from build123d import *

# Parameters (mm, degrees)
SKETCH1_W           = 18
SKETCH1_H           = 3.78
BOSS_EXTRUDE1_DEPTH = 0.5
BOSS_EXTRUDE2_DEPTH = 3.2
SKETCH4_W           = 4
SKETCH4_H           = 3.78
CUT_EXTRUDE1_DEPTH  = 0.8
FILLET1_R           = 4.5


with BuildPart() as part:
    # Sketch1 → Boss-Extrude1 (new body)
    with BuildSketch(Plane.XY):
        Rectangle(SKETCH1_W, SKETCH1_H)
    extrude(amount=BOSS_EXTRUDE1_DEPTH)

    # Sketch3 → Boss-Extrude2 (add)
    with BuildSketch(Plane.XY.offset(0.5)):
        with BuildLine():
            Line((-3.825, -1.89), (3.825, -1.89))
            ThreePointArc((3.825, -1.89), (4.532106781, -1.597106781), (4.825, -0.89))
            Line((4.825, -0.89), (4.825, 0.89))
            ThreePointArc((4.825, 0.89), (4.532106781, 1.597106781), (3.825, 1.89))
            Line((3.825, 1.89), (-3.825, 1.89))
            ThreePointArc((-3.825, 1.89), (-4.532106781, 1.597106781), (-4.825, 0.89))
            Line((-4.825, 0.89), (-4.825, -0.89))
            ThreePointArc((-4.825, -0.89), (-4.532106781, -1.597106781), (-3.825, -1.89))
        make_face()
    extrude(amount=BOSS_EXTRUDE2_DEPTH)

    # Sketch4 → Cut-Extrude1 (cut)
    with BuildSketch(Plane(origin=(0, 0, 0), x_dir=(-1, 0, 0), z_dir=(0, 0, -1))):
        Rectangle(SKETCH4_W, SKETCH4_H)
    extrude(amount=-CUT_EXTRUDE1_DEPTH, mode=Mode.SUBTRACT)

    # Fillet1
    # the kernel refuses this fillet: 4.5 mm, written as the material it takes off along each edge
    with BuildSketch(Plane(origin=(-2, -8.293124237, 0), x_dir=(-1, 0, 0), z_dir=(0, 1, 0))) as fillet1_piece_1:
        with BuildLine():
            CenterArc((2.561249695, 4.5), FILLET1_R, 235.307869415, 34.692130585)
            Line((0, 0.8), (-0.051224994, 0.726))
            ThreePointArc((-0.051224994, 0.726), (-0.09, 0.4), (-0.09, 0))
            Line((-0.09, 0), (0, -0.09))
            Line((0, -0.09), (2.561249695, -0.09))
            Line((2.561249695, -0.09), (2.561249695, 0))
        make_face()
    extrude(amount=16.586248475, mode=Mode.SUBTRACT)
    with BuildSketch(Plane(origin=(2, 8.293124237, 0), x_dir=(1.0735856648108615e-12, 0, 1.0), z_dir=(0, -1, 0))) as fillet1_piece_2:
        with BuildLine():
            CenterArc((4.5, -2.561249695), FILLET1_R, 145.307869415, 34.692130585)
            Line((0, -2.561249695), (-0.09, -2.561249695))
            Line((-0.09, -2.561249695), (-0.09, 0))
            Line((-0.09, 0), (0, 0.09))
            ThreePointArc((0, 0.09), (0.4, 0.09), (0.726, 0.051224994))
            Line((0.726, 0.051224994), (0.8, 0))
        make_face()
    extrude(amount=16.586248475, mode=Mode.SUBTRACT)


solid = part.part
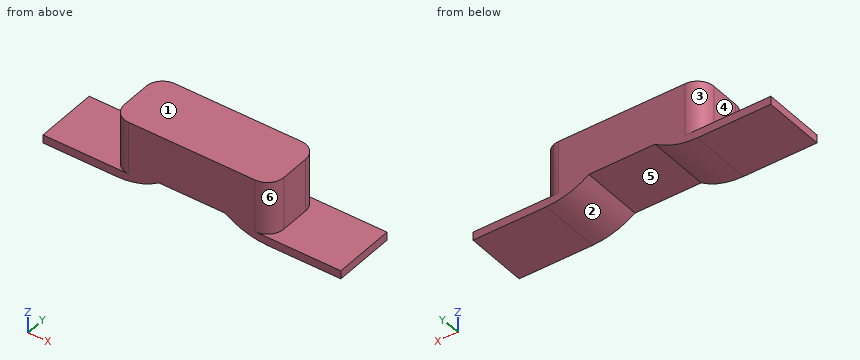
Verification items for the finished model (mm, model axes). Face numbers are marked on the shaded views. A direction names the side the tool comes from. Coordinates: 2 decimals unless noted, no trailing zeros. Order: outer loops, then holes, each group sorted by start corner. A loop starts at its lowest first (then second) coordinate and runs counter-clockwise, first axis right, second up.
Item 1: Access from +Z, -Z, +X, -X, +Y, -Y to the whole of each face (thin tool, end or side, straight path). Record for the marked faces 4, 5 and 6.
Filled in:
face 4: +Z, -X, +Y, -Y
face 5: -Z, +Y, -Y
face 6: +Z, +X, -Y
Item 2: Section check C-C, the plane x = -5.25. Enter the section's corners in (y, z), then the cut area to 3 significant figures.
Filled in:
outline: (-1.89, 0) - (1.89, 0) - (1.89, 0.5) - (-1.89, 0.5) - close
area: 1.89 mm2
Item 3: Section check D-D, the plane y = -1.1. Enter the section's corners in (x, z), then the cut area to 3 significant figures.
Filled in:
outline: (-9, 0) - (-4.56, 0) arc R4.5 ccw to (-2, 0.8) - (2, 0.8) arc R4.5 ccw to (4.56, 0) - (9, 0) - (9, 0.5) - (4.8, 0.5) - (4.8, 3.7) - (-4.8, 3.7) - (-4.8, 0.5) - (-9, 0.5) - close
area: 35.2 mm2
Item 4: Section check A-A, the plane z = 1.7. Enter the section's corners in (x, y) (3 decimals), then the cut area to 3 significant figures.
Filled in:
outline: (-4.825, -0.89) arc R1 ccw to (-3.825, -1.89) - (3.825, -1.89) arc R1 ccw to (4.825, -0.89) - (4.825, 0.89) arc R1 ccw to (3.825, 1.89) - (-3.825, 1.89) arc R1 ccw to (-4.825, 0.89) - close
area: 35.6 mm2
Item 5: Section check B-B, the plane y = 0.3. Enter the section's corners in (x, z) (3 decimals).
Filled in:
outline: (-9, 0) - (-4.561, 0) arc R4.5 ccw to (-2, 0.8) - (2, 0.8) arc R4.5 ccw to (4.561, 0) - (9, 0) - (9, 0.5) - (4.825, 0.5) - (4.825, 3.7) - (-4.825, 3.7) - (-4.825, 0.5) - (-9, 0.5) - close
Item 6: Release check for a two-part mould opening along X. For the marked faces 1, 2 and 3 record: +X half, -X half, draft (parallel to the pull), parting line (faces both ways), or undercut.
Filled in:
face 1: draft
face 2: undercut
face 3: -X half
Item 7: Depth check by flat-ended pin: pin 1 (2 mm diameter, centred on x = -0.5, y = 1.5, fed in from -Z); pin 2 (1.1 mm diameter, centred on x = 6.5, y = 0.5, fed in from +Z); pin 3 (0.9 mm diameter, centred on y = 0, z = 2.5, fed in from -X) (3 decimals). Enter the tip coordinate at first touch or a pass-through.
Filled in:
pin 1: stops at z = 0.8
pin 2: stops at z = 0.5
pin 3: stops at x = -4.825
Item 8: Material ranges on L1, parallel to X at y = -0.25, z = 2.2 (3 decimals); L2, parallel to Z at x = -7.75, y = 0.75; L3, parallel to X at y = 1.05, z = 0.7, recorded low to high.
Filled in:
L1: x = -4.825 to 4.825
L2: z = 0 to 0.5
L3: x = -4.81 to -2.15, 2.15 to 4.81
